Job drawing, mm, ordinate dimensions from the low corner. One solid piece. A direction names the side the tool comes from. Round coordinates to 2 decimals unless told otherwise and drop trailing zeros. Loops run counter-clockwise (first coordinate to the right, second up) from the corner with the lowest first, then second, coordinate; pieces in that order, holes last.
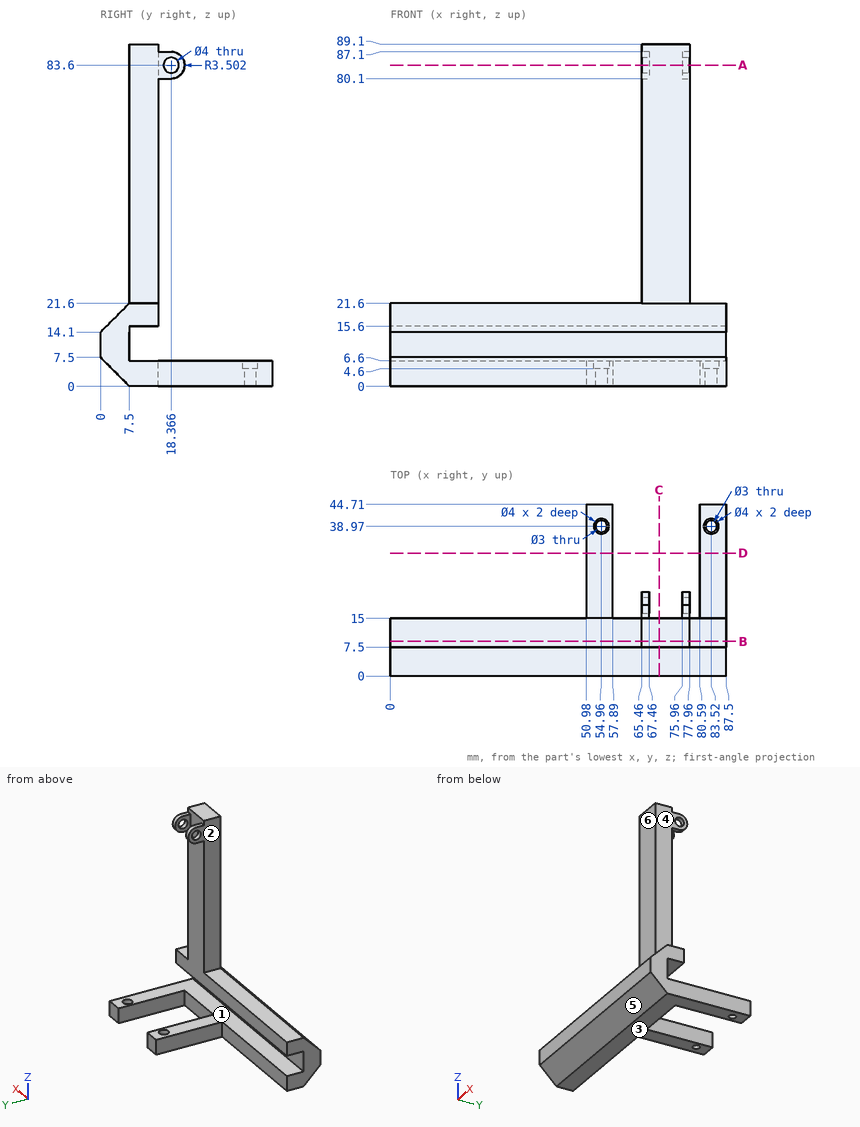
Item 1: Flat gauge pins, fed straight in: P1, Ø10, axis at x = 67.5, z = 66, coming from the +Y side; P2, Ø3.5, axis at y = 34, z = 3, coming from the -X side; P3, Ø1.5, axis at x = 9, y = 8.5, coming from the +Z side. Where does each tip first touch, or does it go through?
Answers follow:
P1: stops at y = 15
P2: stops at x = 50.98
P3: stops at z = 21.6
Item 2: Cut at C-C, the plane x = 70. Give the cut face in (y, z).
Answers follow:
outline: (0, 7.5) - (7.5, 0) - (15, 0) - (15, 6.6) - (7.5, 6.6) - (7.5, 15.6) - (15, 15.6) - (15, 89.1) - (7.5, 89.1) - (7.5, 21.6) - (0, 14.1) - close
Item 3: Cut at A-A, the plane z = 83.6. Give the cut face in (x, y).
Answers follow:
outline: (65.46, 7.5) - (77.96, 7.5) - (77.96, 16.37) - (75.96, 16.37) - (75.96, 15) - (67.46, 15) - (67.46, 16.37) - (65.46, 16.37) - close; (65.46, 20.37) - (67.46, 20.37) - (67.46, 21.87) - (65.46, 21.87) - close; (75.96, 20.37) - (77.96, 20.37) - (77.96, 21.87) - (75.96, 21.87) - close
Item 4: Cut at D-D, the plane y = 32. Give the cut face in (x, z), plus the area to 3 significant figures.
Answers follow:
outline: (50.98, 0) - (57.89, 0) - (57.89, 6.6) - (50.98, 6.6) - close; (80.59, 0) - (87.5, 0) - (87.5, 6.6) - (80.59, 6.6) - close
area: 91.2 mm2
Item 5: 3-axis set-ups, long thin cutter, end or side, ignore diameter. For the marked faces 4, 5 and 6: which of +Z, -Z, +X, -X, +Y, -Y reach the whole face in a straight line?
Answers follow:
face 4: +Z, +X, +Y, -Y
face 5: -Z, +X, -X, -Y
face 6: +Z, +X, -X, -Y
Item 6: Cut at B-B, the plane y = 9. Give the cut face in (x, z).
Answers follow:
outline: (0, 0) - (87.5, 0) - (87.5, 6.6) - (0, 6.6) - close; (0, 15.6) - (87.5, 15.6) - (87.5, 21.6) - (77.96, 21.6) - (77.96, 89.1) - (65.46, 89.1) - (65.46, 21.6) - (0, 21.6) - close
Item 7: Probe line 1 (X direction, y = 20, z = 81.5); line 2 (X direction, y = 29.5, z = 4); line 3 (X direction, y = 8, z = 66). List the from-to ranges inside material, lowest first.
Answers follow:
line 1: x = 65.46 to 67.46, 75.96 to 77.96
line 2: x = 50.98 to 57.89, 80.59 to 87.5
line 3: x = 65.46 to 77.96
Item 8: Two-plate mould, pull along Z, no slides. Class the marked faces 1, 2 and 3: released by +Z, released by -Z, zero draft, split by the parting line, or undercut.
Answers follow:
face 1: undercut
face 2: zero draft
face 3: released by -Z
